from build123d import *

# Parameters (mm, degrees)
PAD_DEPTH    = 20
SKETCH001_W  = 440
SKETCH001_H  = 300
POCKET_DEPTH = 20


with BuildPart() as part:
    # Sketch → Pad (new body)
    with BuildSketch(Plane.YZ):
        Polygon((-220, 475), (220, 475), (320, 375), (320, -375), (220, -475), (-220, -475), (-320, -375), (-320, 375), align=None)
    extrude(amount=PAD_DEPTH)

    # Sketch001 (on Face10 of Pad) → Pocket (cut)
    with BuildSketch(Plane.YZ.offset(20)):
        with Locations((0, 225)):
            Rectangle(SKETCH001_W, SKETCH001_H)
    extrude(amount=-POCKET_DEPTH, mode=Mode.SUBTRACT)


solid = part.part
Part model, mm, in its own coordinate system. A direction names the side the tool comes from. Give positions to 0.01 mm unless a question says otherwise; leave off trailing zeros. Order: outer loops, then holes, each group sorted by start corner. A loop starts at its lowest first (then second) coordinate and runs counter-clockwise, first axis right, second up. Notation, with made-up numbers: (49, 82) - (90, 82) arc R31 ccw to (90, 119) - close; hole circle Ø3 at (10.5, 14.5). An arc over 180 degrees is marked (long way). Use a Markdown table: item, result.
1) 3-axis set-ups, long thin cutter, end or side, ignore diameter. For faces 1 (the flat face through (10, 269, 426)), 2 (the flat face through (10, -3, 375)): which of +Z, -Z, +X, -X, +Y, -Y reach the whole face in a straight line?
Checked values:
| item | result |
|---|---|
| face 1 | +Z, +X, -X, +Y |
| face 2 | +X, -X |
2) Saw through at A-A on z = 270.5. List the corners of the cut face in (x, y).
Checked values:
| item | result |
|---|---|
| outline | (0, -320) - (20, -320) - (20, -220) - (0, -220) - close; (0, 220) - (20, 220) - (20, 320) - (0, 320) - close |
3) Saw through at B-B on y = 17. List the corners of the cut face in (x, z), plus the area to 3 significant figures.
Checked values:
| item | result |
|---|---|
| outline | (0, -475) - (20, -475) - (20, 75) - (0, 75) - close; (0, 375) - (20, 375) - (20, 475) - (0, 475) - close |
| area | 13,000 mm² |
4) Saw through at C-C on x = 5.25. List the corners of the cut face in (y, z).
Checked values:
| item | result |
|---|---|
| outline | (-320, -375) - (-220, -475) - (220, -475) - (320, -375) - (320, 375) - (220, 475) - (-220, 475) - (-320, 375) - close; hole (-220, 75) - (220, 75) - (220, 375) - (-220, 375) - close |
5) Probe L1, parallel to Y at x = 8.5, z = 278.5; L2, parallel to Z at x = 8.75, y = 87; L3, parallel to Y at x = 10.5, z = -379. List the from-to ranges inside material, lowest first. Write a range as from..to.
Checked values:
| item | result |
|---|---|
| L1 | -320..-220, 220..320 |
| L2 | -475..75, 375..475 |
| L3 | -316..316 |
6) Saw through at D-D on z = 407. List the corners of the cut face in (x, y), plus the area to 3 significant figures.
Checked values:
| item | result |
|---|---|
| outline | (0, -288) - (20, -288) - (20, 288) - (0, 288) - close |
| area | 11,500 mm² |
7) Two-plate mould, pull along Y, no slides. Class faces 3 (the flat face through (10, 220, 223)), 4 (the flat face through (10, -269, -426)), 5 (the flat face through (10, -3, 475)): +Y half, -Y half, draft (parallel to the pull), parting line (faces both ways), or undercut.
Checked values:
| item | result |
|---|---|
| face 3 | undercut |
| face 4 | -Y half |
| face 5 | draft |
